from build123d import *

# Parameters (mm, degrees)
CHAMFER1_SIZE = 1.5


with BuildPart() as part:
    # Sketch1 → Revolve1 (revolve)
    with BuildSketch(Plane.XY, mode=Mode.PRIVATE) as revolve1_sk:
        with BuildLine():
            Line((0, 0), (0, 85.55))
            Line((0, 85.55), (3.18, 85.55))
            Line((3.18, 85.55), (3.18, 15.766075305))
            ThreePointArc((3.18, 15.766075305), (10.355139161, 3.27502159), (24.76, 3.18))
            Line((24.76, 3.18), (26.67, 1.27))
            Line((26.67, 1.27), (26.67, 0))
            Line((26.67, 0), (0, 0))
        make_face()
    revolve(revolve1_sk.sketch.rotate(Axis((0, 0, 0), (0, 1, 0)), 90), axis=Axis((0, 0, 0), (0, 1, 0)))

    # Chamfer1
    chamfer1_edges = [part.edges().sort_by_distance(p)[0] for p in [
        (0, 85.55, 3.18),
    ]]
    chamfer(chamfer1_edges, length=CHAMFER1_SIZE)


solid = part.part
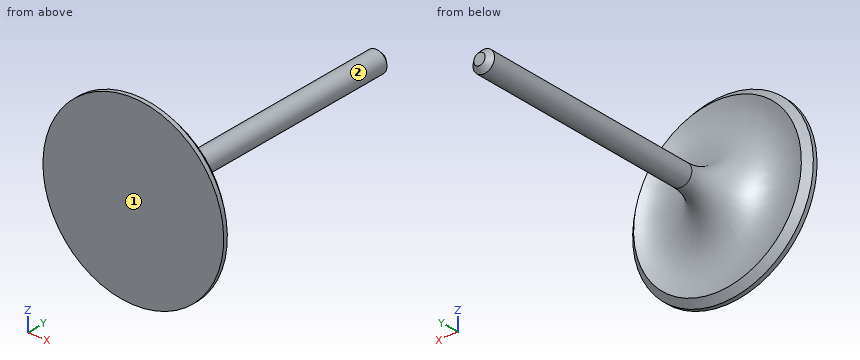
The listing builds one solid part. Answer for the finished solid, in the listing's coordinates (mm). Face numbers are marked on the shaded views. A direction names the side the tool comes from. Round coordinates to 2 decimals unless told otherwise and drop trailing zeros. Write each loop counter-clockwise with the first axis right and the second up, starting at its lowest first coordinate (ties: lowest second). Pieces come first, ordered by that corner, then holes. Notation, with made-up numbers: (32.25, 80.25) - (87.25, 80.25) arc R20 cw to (87.25, 88.25) - close; hole circle Ø7 at (78, 77.25). An arc over 180 degrees is marked (long way). Use one line per item in the form item = value. Start each with the question number.
Item 1: Find the intervals of material crossed by line 1 (Y direction, x = 3, z = 17); line 2 (X direction, y = 78, z = 2.5); line 3 (Y direction, x = -20, z = 2), in increasing order. Write a range as [from, to].
Item 2: A tool of negligible diameter and unlimited length cuts with its end or side. For the marked faces 1 and 2, from which of +Z, -Z, +X, -X, +Y, -Y can it reach the whole face along a straight path? Write none if from no direction.
Item 3: A cutting plane is placed at C-C (y = 55.5). Write down the section's boundary in (x, z).
Item 4: Flat-ended cylindrical pins translate along their axes: pin 1 Ø3 at (x, z) = (8, -10.5) entering from +Y; pin 2 Ø2 at (x, z) = (-0.5, -4) entering from +Y; pin 3 Ø4 at (x, z) = (17.5, 5.5) entering from +Y. Find the tip coordinate at first contact, or state that the pin passes through.
Item 5: A cutting plane is placed at A-A (z = 0). Write down the section's boundary in (x, y), plus the area to 3 significant figures.
Item 6: A cutting plane is placed at B-B (x = 0). Write down the section's boundary in (y, z).
The answers:
q1.line_1 = [0, 1.31]
q1.line_2 = [-1.97, 1.97]
q1.line_3 = [0, 1.52]
q2.face_1 = +Z, -Z, +X, -X, -Y
q2.face_2 = +Y
q3.outline = circle Ø6.36 at (0, 0)
q4.pin_1 = 2.58
q4.pin_2 = 84.2
q4.pin_3 = 1.56
q5.outline = (-26.67, 0) - (26.67, 0) - (26.67, 1.27) - (24.76, 3.18) arc R14.46 cw to (3.18, 15.77) - (3.18, 84.05) - (1.68, 85.55) - (-1.68, 85.55) - (-3.18, 84.05) - (-3.18, 15.77) arc R14.46 cw to (-24.76, 3.18) - (-26.67, 1.27) - close
q5.area = 705 mm^2
q6.outline = (0, -26.67) - (1.27, -26.67) - (3.18, -24.76) arc R14.46 cw to (15.77, -3.18) - (84.05, -3.18) - (85.55, -1.68) - (85.55, 1.68) - (84.05, 3.18) - (15.77, 3.18) arc R14.46 cw to (3.18, 24.76) - (1.27, 26.67) - (0, 26.67) - close
